from build123d import *

# Parameters (mm, degrees)
SKETCH2_W           = 40
SKETCH2_H           = 40
BOSS_EXTRUDE1_DEPTH = 20
SKETCH3_W           = 20
SKETCH3_H           = 10
CUT_EXTRUDE1_DEPTH  = 20
SKETCH6_R           = 10
BOSS_EXTRUDE2_DEPTH = 20


with BuildPart() as part:
    # Sketch2 → Boss-Extrude1 (new body)
    with BuildSketch(Plane(origin=(0, 0, 0), x_dir=(1, 0, 0), z_dir=(0, 1, 0))):
        with Locations((20, 20)):
            Rectangle(SKETCH2_W, SKETCH2_H)
    extrude(amount=BOSS_EXTRUDE1_DEPTH)

    # Sketch3 → Cut-Extrude1 (cut)
    with BuildSketch(Plane.XY):
        with Locations((20, 5)):
            Rectangle(SKETCH3_W, SKETCH3_H)
    extrude(amount=-CUT_EXTRUDE1_DEPTH, mode=Mode.SUBTRACT)

    # Sketch6 → Boss-Extrude2 (add)
    with BuildSketch(Plane(origin=(0, 20, 0), x_dir=(1, 0, 0), z_dir=(0, 1, 0))):
        with Locations(Location((20, 21.579352737, 0), (0, 0, 270))):
            Circle(SKETCH6_R)
    extrude(amount=BOSS_EXTRUDE2_DEPTH)


solid = part.part
Could you check a few things on this model? Use its own coordinates, in mm. A direction names the side the tool comes from. Give positions to 0.01 mm unless a question says otherwise; leave off trailing zeros. Order: outer loops, then holes, each group sorted by start corner. A loop starts at its lowest first (then second) coordinate and runs counter-clockwise, first axis right, second up.
1. Suppose I cut it at A-A (y = 3). Write out the boundary of the cut face in (x, z), plus the area to 3 significant figures.
Answers below:
outline: (0, -40) - (40, -40) - (40, 0) - (30, 0) - (30, -20) - (10, -20) - (10, 0) - (0, 0) - close
area: 1,200 mm2
2. Thinking about a two-plate mould opening in X: for faces 4 (the flat face through (20, 10, -40)), 5 (the flat face through (20, 10, -10)), 6 (the flat face through (0, 10, -20)), 7 (the flat face through (10, 5, -10)), which applies, +X half, -X half, draft (parallel to the pull), parting line (faces both ways), or undercut?
Answers below:
face 4: draft
face 5: undercut
face 6: -X half
face 7: undercut
3. Which directions (+Z, -Z, +X, -X, +Y, -Y) give clear straight access to the entire face, cutting with the end or side of a thin tool? Please do faces 1 (the flat face through (20, 20, -11)), 2 (the flat face through (30, 5, -10)), 3 (the flat face through (20, 0, -25)).
Answers below:
face 1: +Y
face 2: +Z, -Y
face 3: +Z, -Z, +X, -X, -Y
4. Suppose I cut it at B-B (x = 20). Write out the boundary of the cut face in (y, z).
Answers below:
outline: (0, -40) - (20, -40) - (20, -31.58) - (40, -31.58) - (40, -11.58) - (20, -11.58) - (20, 0) - (10, 0) - (10, -20) - (0, -20) - close
5. Suppose I cut it at D-D (x = 16). Write out the boundary of the cut face in (y, z).
Answers below:
outline: (0, -40) - (20, -40) - (20, -30.74) - (40, -30.74) - (40, -12.41) - (20, -12.41) - (20, 0) - (10, 0) - (10, -20) - (0, -20) - close
6. I need wall thicknesses on L1, parallel to X at y = 3.5, z = -7.5; L2, parallel to Y at x = 17, z = -8; L3, parallel to Y at x = 20, z = -15. Which ranges of each line are inside material? Lowest first, please.
Answers below:
L1: x = 0 to 10, 30 to 40
L2: y = 10 to 20
L3: y = 10 to 40
7. For pin 1 (5 mm diameter, centred on x = 7, y = 28, fed in from -Z); pin 2 (6 mm diameter, centred on y = 35.5, z = -13, fed in from +X), each with a flat end and sliding along its axis, tell me the tip position at first contact or that it passes through.
Answers below:
pin 1: passes through
pin 2: stops at x = 28.3
8. Suppose I cut it at C-C (z = -15). Write out the boundary of the cut face in (x, y).
Answers below:
outline: (0, 0) - (10, 0) - (10, 10) - (30, 10) - (30, 0) - (40, 0) - (40, 20) - (27.53, 20) - (27.53, 40) - (12.47, 40) - (12.47, 20) - (0, 20) - close
